```python
from build123d import *

# Parameters (mm, degrees)
F0_W      = 45
F0_H      = 80
F1_DEPTH  = 7
F2_R      = 5
F4_DEPTH  = 8
F5_R      = 3.4
F6_DEPTH  = 8.5
F7_W      = 4
F7_H      = 0.8
F8_DEPTH  = 26
F9_W      = 6.5
F9_H      = 0.8
F10_DEPTH = 26
F11_W     = 7
F11_H     = 0.8
F12_DEPTH = 26
F13_W     = 10
F13_H     = 1
F14_DEPTH = 20.5
F15_R     = 4
F16_DEPTH = 0.2
F17_W     = 40
F17_H     = 58
F18_DEPTH = 0.1


with BuildPart() as f1:
    # F0 (on Top) → F1 (new body)
    with BuildSketch(Plane.XY):
        with Locations((2.694569, -2.665429)):
            Rectangle(F0_W, F0_H)
    extrude(amount=F1_DEPTH)

    # F2
    f2_edges = [f1.edges().sort_by_distance(p)[0] for p in [
        (-19.805431, 37.334571, 3.5),
        (25.194569, 37.334571, 3.5),
        (-19.805431, -42.665429, 3.5),
        (25.194569, -42.665429, 3.5),
    ]]
    fillet(f2_edges, radius=F2_R)

    # F3 (on Top) → F4 (join)
    with BuildSketch(Plane.XY):
        with BuildLine():
            Line((-3.5, 34.334571), (-12.5, 34.334571))
            ThreePointArc((-12.5, 34.334571), (-14.974874, 33.309444), (-16, 30.834571))
            ThreePointArc((-16, 30.834571), (-14.974874, 28.359697), (-12.5, 27.334571))
            Line((-12.5, 27.334571), (-3.5, 27.334571))
            ThreePointArc((-3.5, 27.334571), (-1.025126, 28.359697), (0, 30.834571))
            ThreePointArc((0, 30.834571), (-1.025126, 33.309444), (-3.5, 34.334571))
        make_face()
    extrude(amount=F4_DEPTH)

    # F5 (on Top) → F6 (join)
    with BuildSketch(Plane.XY):
        with Locations((-12.527948, 30.834571)):
            Circle(F5_R)
    extrude(amount=F6_DEPTH)

    # F7 (on Right) → F8 (join)
    with BuildSketch(Plane.YZ):
        with Locations((26.334571, 3.018534)):
            Rectangle(F7_W, F7_H)
    extrude(amount=F8_DEPTH)

    # F9 (on Right) → F10 (join)
    with BuildSketch(Plane.YZ):
        with Locations((18.387751, 3)):
            Rectangle(F9_W, F9_H)
    extrude(amount=F10_DEPTH)

    # F11 (on Right) → F12 (join)
    with BuildSketch(Plane.YZ):
        with Locations((9.535096, 3)):
            Rectangle(F11_W, F11_H)
    extrude(amount=F12_DEPTH)

    # F13 (on Right) → F14 (join)
    with BuildSketch(Plane.YZ):
        with Locations((15.474138, 3.5)):
            Rectangle(F13_W, F13_H)
    extrude(amount=-F14_DEPTH)

    # F15 (on Top) → F16 (join)
    with BuildSketch(Plane.XY):
        with Locations((2.694569, -35.592675)):
            Circle(F15_R)
    extrude(amount=-F16_DEPTH)

    # F17 (on Top) → F18 (join)
    with BuildSketch(Plane.XY):
        with Locations((2.694569, 0.584052)):
            Rectangle(F17_W, F17_H)
    extrude(amount=-F18_DEPTH)


solid = f1.part
```
Check sheet for the modelled part. Datum: model origin and axes. Units: mm. A direction names the side the tool comes from. Coordinates: 2 decimals unless noted, no trailing zeros. Order: outer loops, then holes, each group sorted by start corner. A loop starts at its lowest first (then second) coordinate and runs counter-clockwise, first axis right, second up. Notation, with made-up numbers: (37.25, 7.5) -> (55.25, 7.5) arc R29 ccw to (55.25, 30.5) -> close; hole circle Ø1 at (10, -25). An arc over 180 degrees is marked (long way). Write item = value, one per line. Start each with the question number.
1) Cross-section at C-C (y = 16). Enter the section's corners in (x, z).
2) Material ranges on L1, parallel to Z at x = 15, y = 9.5; L2, parallel to Z at x = 8.5, y = -39; L3, parallel to X at y = 18, z = 3.5, recorded low to high.
3) Cross-section at A-A (x = 10.5). Enter the section's corners in (y, z), then the cut area to 3 significant figures.
4) Cross-section at D-D (x = -11.5). Enter the section's corners in (y, z).
5) Go/stop test with flat-tipped pins: P1, Ø3, axis at y = 13, z = 5.5, coming from the +X side; P2, Ø3, axis at x = -7, y = -12.5, coming from the -Z side; P3, Ø0.9, axis at x = 26, z = 3, coming from the -Y side. Record where each tip stops, or that it passes through.
6) Access from +Z, -Z, +X, -X, +Y, -Y to the whole of each face (thin tool, end or side, straight path). Record for faces 1 (the flat face through (2, 37.335, 3)), 2 (the cylindrical face through (-10.959, 27.818, 8.246)).
7) Cross-section at B-B (y = -17). Enter the section's corners in (x, z), then the cut area to 3 significant figures.
Ans:
q1.outline = (-20.5, 3) -> (-19.81, 3) -> (-19.81, 0) -> (-17.31, 0) -> (-17.31, -0.1) -> (22.69, -0.1) -> (22.69, 0) -> (25.19, 0) -> (25.19, 2.6) -> (26, 2.6) -> (26, 3.4) -> (25.19, 3.4) -> (25.19, 7) -> (-19.81, 7) -> (-19.81, 4) -> (-20.5, 4) -> close
q2.L1 = -0.1 to 7
q2.L2 = 0 to 7
q2.L3 = -20.5 to 25.19
q3.outline = (-42.67, 0) -> (-28.42, 0) -> (-28.42, -0.1) -> (29.58, -0.1) -> (29.58, 0) -> (37.33, 0) -> (37.33, 7) -> (-42.67, 7) -> close
q3.area = 566 mm²
q4.outline = (-42.67, 0) -> (-28.42, 0) -> (-28.42, -0.1) -> (29.58, -0.1) -> (29.58, 0) -> (37.33, 0) -> (37.33, 7) -> (34.33, 7) -> (34.33, 8) -> (34.08, 8) -> (34.08, 8.5) -> (27.59, 8.5) -> (27.59, 8) -> (27.33, 8) -> (27.33, 7) -> (-42.67, 7) -> close
q5.P1 = 25.19
q5.P2 = -0.1
q5.P3 = 6.04
q6.face_1 = +Z, -Z, +X, -X, +Y
q6.face_2 = +Z
q7.outline = (-19.81, 0) -> (-17.31, 0) -> (-17.31, -0.1) -> (22.69, -0.1) -> (22.69, 0) -> (25.19, 0) -> (25.19, 7) -> (-19.81, 7) -> close
q7.area = 319 mm²
